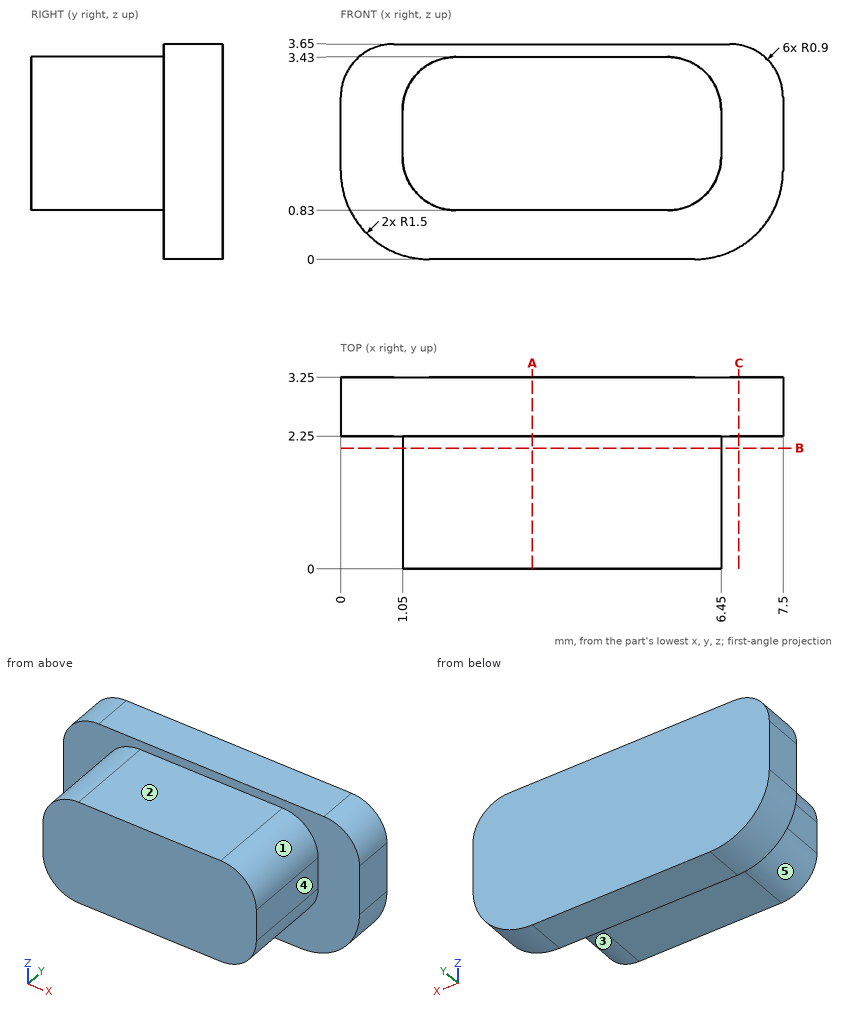
Here's the drawing with two shaded views (mm, measured from the low corner). I have some questions. A direction names the side the tool comes from. Give positions to 0.01 mm unless a question says otherwise; leave off trailing zeros. Loops run counter-clockwise (first coordinate to the right, second up) from the corner with the lowest first, then second, coordinate; pieces in that order, holes last. Notation, with made-up numbers: (41, -15.75) -> (97, -15.75) arc R20 cw to (97, 5.25) -> close; hole circle Ø2 at (-16.5, 19.5). An arc over 180 degrees is marked (long way). Answer as a JSON object with one key per item and string values. Group by question number.
Item 1: Will this pin go through, and if not, where does the flat tip stop? pin 1 (0.7 mm diameter, centred on x = 4, y = 1, fed in from -Z).
Item 2: Imagine slicing it at A-A on x = 3.25. Write out the boundary of the cut face in (y, z), then the cut area to 3 significant figures.
Item 3: Imagine slicing it at C-C on x = 6.75. Write out the boundary of the cut face in (y, z).
Item 4: Imagine slicing it at B-B on y = 2.05. Write out the boundary of the cut face in (x, z).
Item 5: On a 3-axis mill with a long thin cutter (end or side, diameter ignored), from which of +Z, -Z, +X, -X, +Y, -Y can I reach the whole of each face in a straight line? I mean the marked faces 1, 2, 3, 4 and 5. Say none if no direction works.
Item 6: I need wall thicknesses on L1, parallel to Z at x = 3, y = 2.1; L2, parallel to Y at x = 6.5, z = 1.25; L3, parallel to X at y = 2.05, z = 1.8. Which ranges of each line are inside material? Lowest first, please.
Answer list:
{
 "1": {"pin 1": "stops at z = 0.83"},
 "2": {"outline": "(0, 0.83) -> (2.25, 0.83) -> (2.25, 0) -> (3.25, 0) -> (3.25, 3.65) -> (2.25, 3.65) -> (2.25, 3.43) -> (0, 3.43) -> close", "area": "9.50 mm2"},
 "3": {"outline": "(2.25, 0.2) -> (3.25, 0.2) -> (3.25, 3.64) -> (2.25, 3.64) -> close"},
 "4": {"outline": "(1.05, 1.73) arc R0.9 ccw to (1.95, 0.83) -> (5.55, 0.83) arc R0.9 ccw to (6.45, 1.73) -> (6.45, 2.53) arc R0.9 ccw to (5.55, 3.43) -> (1.95, 3.43) arc R0.9 ccw to (1.05, 2.53) -> close"},
 "5": {"face 1": "+Z, +X, -Y", "face 2": "+Z, +X, -X, -Y", "face 3": "-Z, +X, -Y", "face 4": "+Z, -Z, +X, -Y", "face 5": "-Z, -X, -Y"},
 "6": {"L1": "z = 0.83 to 3.43", "L2": "y = 2.25 to 3.25", "L3": "x = 1.05 to 6.45"}
}
